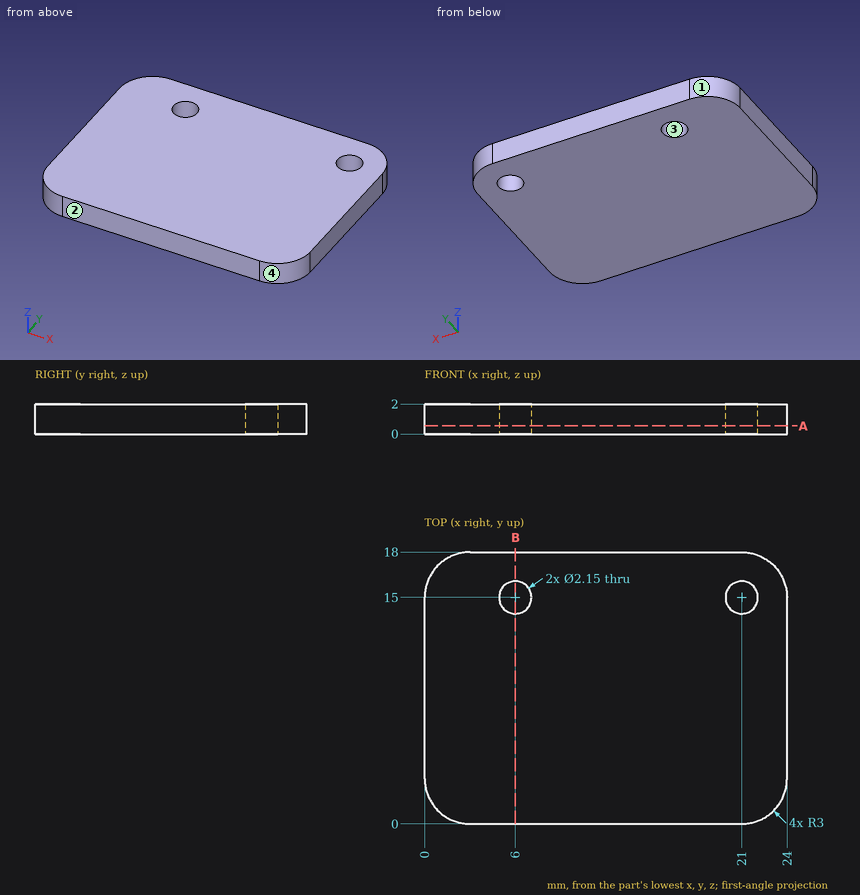
Geometry: see drawing. Coordinates: mm, zero at the bounding-box minimum. Give positions to 0.01 mm unless a question says otherwise; leave off trailing zeros. Order: outer loops, then holes, each group sorted by start corner. A loop starts at its lowest first (then second) coordinate and runs counter-clockwise, first axis right, second up.
Q1. Section B-B on x = 6. Output: boundary loops of the cut face in (y, z) (3 decimals), and give its area (3 significant figures).
Checked values:
outline: (0, 0) - (13.925, 0) - (13.925, 2) - (0, 2) - close; (16.075, 0) - (18, 0) - (18, 2) - (16.075, 2) - close
area: 31.7 mm2
Q2. Ray query, probe 1 along Y at (x, z) = (6, 0.8) (3 decimals); probe 2 along Y at (x, z) = (5.75, 1.2); probe 3 along Y at (x, z) = (2.25, 0.8). Return the intervals inside material, ascending.
Checked values:
probe 1: y = 0 to 13.925, 16.075 to 18
probe 2: y = 0 to 13.95, 16.05 to 18
probe 3: y = 0.1 to 17.9
Q3. Section A-A on z = 0.55. Output: boundary loops of the cut face in (x, y) (3 decimals), and give its area (3 significant figures).
Checked values:
outline: (0, 3) arc R3 ccw to (3, 0) - (21, 0) arc R3 ccw to (24, 3) - (24, 15) arc R3 ccw to (21, 18) - (3, 18) arc R3 ccw to (0, 15) - close; hole circle Ø2.15 at (6, 15); hole circle Ø2.15 at (21, 15)
area: 417 mm2
Q4. Contact query for a flat-ended pin moving along its axis: pin 1 Ø3 at (x, y) = (6, 15) entering from +Z. Output: stop coordinate, or through.
Checked values:
pin 1: stops at z = 2
Q5. Draft query along X for the marked faces 1, 2, 3 and 4. Return one class per face: +X half, -X half, draft (parallel to the pull), parting line (faces both ways), or undercut.
Checked values:
face 1: -X half
face 2: draft
face 3: undercut
face 4: +X half
